from build123d import *

# Parameters (mm, degrees)
SKETCH_1_W              = 80
SKETCH_1_H              = 62
EXTRUDE_1_DEPTH         = 3
HOLE_WIZARD_4_0_4_1_D   = 4
HOLE_WIZARD_3_2_3_2_1_D = 3.2
CUT_EXTRUDE_1_DEPTH     = 3
HOLE_WIZARD_3_0_3_1_D   = 3
FILLET_1_R              = 5


with BuildPart() as part:
    # 草图1 → 凸台-拉伸1 (new body)
    with BuildSketch(Plane.XY):
        with Locations((-2.5, 0)):
            Rectangle(SKETCH_1_W, SKETCH_1_H)
    extrude(amount=EXTRUDE_1_DEPTH)

    # Ø4.0 (4) 直径孔1 (through all)
    with Locations(Plane.XY.offset(3)):
        with Locations((27.5, 21), (-32.5, 21)):
            Hole(HOLE_WIZARD_4_0_4_1_D / 2)

    # Ø3.2 (3.2) 直径孔1 (through all)
    with Locations(Plane.XY.offset(3)):
        with Locations((14.5, -4.4), (4.5, -4.4)):
            Hole(HOLE_WIZARD_3_2_3_2_1_D / 2)

    # 草图6 → 切除-拉伸1 (cut)
    with BuildSketch(Plane.XY.offset(3)):
        Polygon((-42.5, 11), (-42.5, -31), (-12.5, -31), align=None)
    extrude(amount=-CUT_EXTRUDE_1_DEPTH, mode=Mode.SUBTRACT)

    # Ø3.0 (3) 直径孔1 (through all)
    with Locations(Plane.XY.offset(3)):
        with Locations((27.5, -23.5), (-0.5, -23.5)):
            Hole(HOLE_WIZARD_3_0_3_1_D / 2)

    # 圆角1
    fillet_1_edges = [part.edges().sort_by_distance(p)[0] for p in [
        (-42.5, 11, 1.5),
        (-12.5, -31, 1.5),
        (37.5, -31, 1.5),
        (-42.5, 31, 1.5),
        (37.5, 31, 1.5),
    ]]
    fillet(fillet_1_edges, radius=FILLET_1_R)


solid = part.part
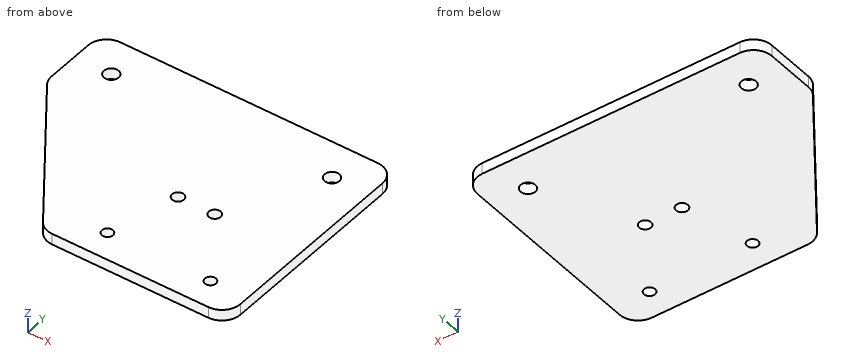
Geometry check sheet. Reference: the model listing, model coordinates, mm. Give positions to 0.01 mm unless a question says otherwise; leave off trailing zeros. Order: outer loops, then holes, each group sorted by start corner. A loop starts at its lowest first (then second) coordinate and runs counter-clockwise, first axis right, second up.
1. Sectioned sample at D-D (y = -4.4). Record the boundary of the cut face in (x, z), then the cut area to 3 significant figures.
Completed:
outline: (-31.5, 0) - (2.9, 0) - (2.9, 3) - (-31.5, 3) - close; (6.1, 0) - (12.9, 0) - (12.9, 3) - (6.1, 3) - close; (16.1, 0) - (37.5, 0) - (37.5, 3) - (16.1, 3) - close
area: 188 mm2
2. Sectioned sample at C-C (z = 2.25). Record the boundary of the cut face in (x, y), then the cut area to 3 significant figures.
Completed:
outline: (-42.5, 12.6) arc R5 ccw to (-41.57, 9.7) - (-14, -28.91) arc R5 ccw to (-9.93, -31) - (32.5, -31) arc R5 ccw to (37.5, -26) - (37.5, 26) arc R5 ccw to (32.5, 31) - (-37.5, 31) arc R5 ccw to (-42.5, 26) - close; hole circle Ø4 at (-32.5, 21); hole circle Ø3 at (-0.5, -23.5); hole circle Ø3.2 at (4.5, -4.4); hole circle Ø3.2 at (14.5, -4.4); hole circle Ø4 at (27.5, 21); hole circle Ø3 at (27.5, -23.5)
area: 4,260 mm2
3. Sectioned sample at A-A (y = 21). Record the boundary of the cut face in (x, z).
Completed:
outline: (-42.5, 0) - (-34.5, 0) - (-34.5, 3) - (-42.5, 3) - close; (-30.5, 0) - (25.5, 0) - (25.5, 3) - (-30.5, 3) - close; (29.5, 0) - (37.5, 0) - (37.5, 3) - (29.5, 3) - close
4. Sectioned sample at B-B (x = 4.5). Record the boundary of the cut face in (y, z), then the cut area to 3 significant figures.
Completed:
outline: (-31, 0) - (-6, 0) - (-6, 3) - (-31, 3) - close; (-2.8, 0) - (31, 0) - (31, 3) - (-2.8, 3) - close
area: 176 mm2
5. Scan lines: line 1 (Y direction, x = 27.5, z = 2.35); line 2 (Y direction, x = 14.5, z = 2.45); line 3 (Y direction, x = -0.5, z = 2.15). Record each from-to range of solid material in increasing order.
Completed:
line 1: y = -31 to -25, -22 to 19, 23 to 31
line 2: y = -31 to -6, -2.8 to 31
line 3: y = -31 to -25, -22 to 31
6. Depth check by flat-ended pin: pin 1 (4 mm diameter, centred on x = 4.5, y = -4.4, fed in from +Z). Enter the tip coordinate at first touch or a pass-through.
Completed:
pin 1: stops at z = 3
